Design review of the part shown in the three views and the two pictorial views. Dimensions are in mm from the part's minimum x, y and z. A direction names the side the tool comes from. Coordinates: 2 decimals unless noted, no trailing zeros. Loops run counter-clockwise (first coordinate to the right, second up) from the corner with the lowest first, then second, coordinate; pieces in that order, holes last. Notation, with made-up numbers: M 60,63.5 L 112,63.5 A19 ccw 112,97.5 Z; hole C 4,43.25 d4. An arc over 180 degrees is marked long. Put each result on its own line as item: value. Start each with the question number.
(1) Take a section at C-C, the plane y = 38.1. Give the boundary of the cut face in (x, z).
(2) Take a section at A-A, the plane z = 38.1. Give the boundary of the cut face in (x, y).
(3) For probe 1 along X at (y, z) = (95, 38.1); probe 2 along X at (y, z) = (35, 19.5); probe 3 along Z at (x, y) = (97, 121), list the stretches that pass through material, from the lowest coordinate up. Write a range as [from, to].
(4) For the marked faces 1, 2 and 3, list the 3-axis set-ups (+Z, -Z, +X, -X, +Y, -Y) from which the entire face can be reached by the end or side of a thin tool; tool diameter is ignored.
(5) Clearance check with flat-ended pins moving along their axes: pin 1 (23 mm diameter, centred on y = 65, z = 45, fed in from -X); pin 2 (8.5 mm diameter, centred on x = 93, z = 34.5, fed in from +Y); pin 3 (1 mm diameter, centred on x = 22, z = 42.5, fed in from -Y); pin 4 (4 mm diameter, centred on x = 85.5, y = 23.5, fed in from -Z). State where each tip first meets the part, or that it passes through.
(6) Take a section at B-B, the plane x = 88.9. Give the boundary of the cut face in (y, z).
(7) Take a section at D-D, the plane z = 8.5. Give the boundary of the cut face in (x, y), then the cut area to 3 significant figures.
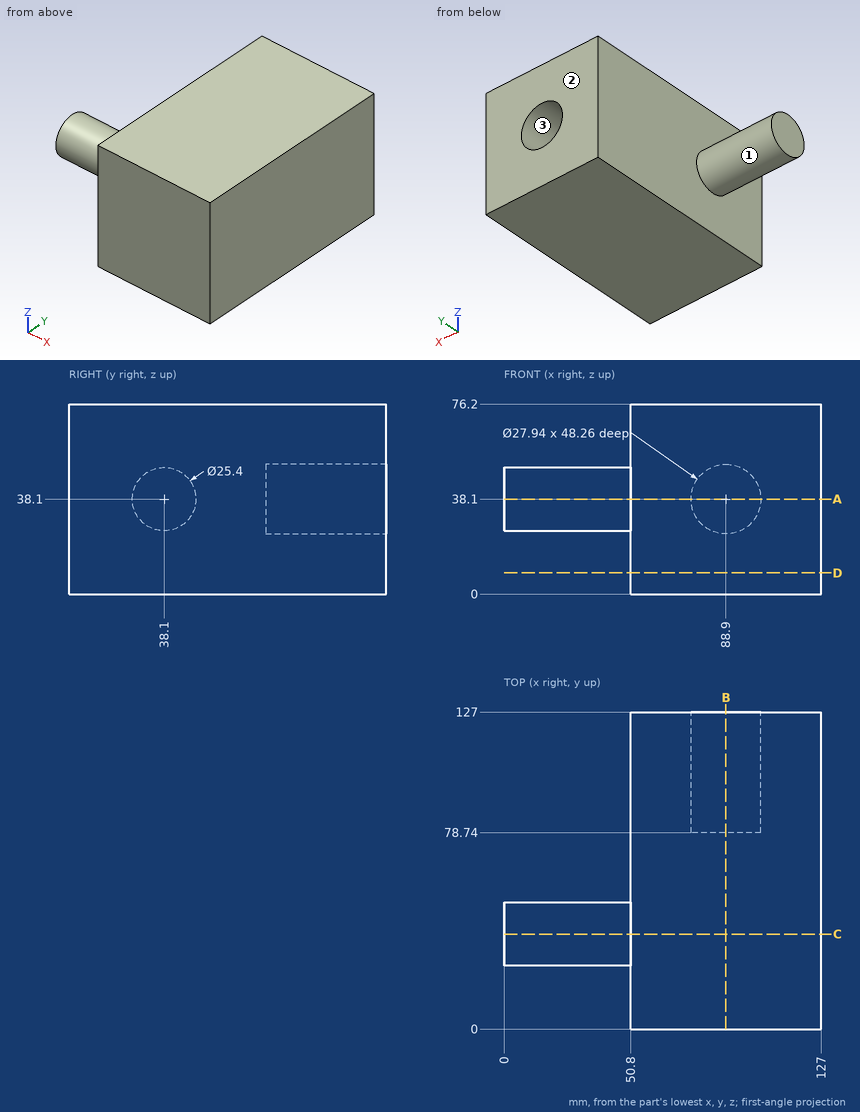
Computed values:
1. outline: M 0,25.4 L 50.8,25.4 L 50.8,0 L 127,0 L 127,76.2 L 50.8,76.2 L 50.8,50.8 L 0,50.8 Z
2. outline: M 0,25.4 L 50.8,25.4 L 50.8,0 L 127,0 L 127,127 L 102.87,127 L 102.87,78.74 L 74.93,78.74 L 74.93,127 L 50.8,127 L 50.8,50.8 L 0,50.8 Z
3. probe 1: x = [50.8, 74.93], [102.87, 127]
3. probe 2: x = [50.8, 127]
3. probe 3: z = [0, 26.72], [49.48, 76.2]
4. face 1: -X
4. face 2: +Z, -Z, +X, -X, +Y
4. face 3: +Y
5. pin 1: stops at x = 50.8
5. pin 2: stops at y = 78.74
5. pin 3: stops at y = 26.01
5. pin 4: stops at z = 0
6. outline: M 0,0 L 127,0 L 127,24.13 L 78.74,24.13 L 78.74,52.07 L 127,52.07 L 127,76.2 L 0,76.2 Z
7. outline: M 50.8,0 L 127,0 L 127,127 L 50.8,127 Z
7. area: 9,680 mm^2
